Read the model definition and answer for the solid it produces. Units are mm, in the model's axes. A direction names the side the tool comes from. Coordinates: 2 decimals unless noted, no trailing zeros. Order: outer loops, then holes, each group sorted by start corner. A loop starts at its lowest first (then second) coordinate and runs counter-clockwise, first axis right, second up. Notation, with made-up numbers: (32.5, -2) -> (65.5, -2) arc R20 cw to (65.5, 23) -> close; hole circle Ø6 at (88.25, 57). An arc over 180 degrees is marked (long way). Answer in a Markdown table with one row per item.
from build123d import *

# Parameters (mm, degrees)
SKETCH1_R           = 28.575
SKETCH1_R_2         = 2.54
BOSS_EXTRUDE1_DEPTH = 4.064
SKETCH2_R           = 14.2875
BOSS_EXTRUDE2_DEPTH = 0.8636
SKETCH3_R           = 12.065
EXTRUDE_M_DEPTH     = 20.4724


with BuildPart() as part:
    # Sketch1 → Boss-Extrude1 (new body)
    with BuildSketch(Plane.XY):
        Circle(SKETCH1_R)
        with Locations((0, 23.8125)):
            Circle(SKETCH1_R_2, mode=Mode.SUBTRACT)
        with Locations((20.622229928, 11.90625)):
            Circle(SKETCH1_R_2, mode=Mode.SUBTRACT)
        with Locations((20.622229928, -11.90625)):
            Circle(SKETCH1_R_2, mode=Mode.SUBTRACT)
        with Locations((0, -23.8125)):
            Circle(SKETCH1_R_2, mode=Mode.SUBTRACT)
        with Locations((-20.622229928, -11.90625)):
            Circle(SKETCH1_R_2, mode=Mode.SUBTRACT)
        with Locations((-20.622229928, 11.90625)):
            Circle(SKETCH1_R_2, mode=Mode.SUBTRACT)
        Polygon((7.332348419, 0), (3.666174209, 6.35), (-3.666174209, 6.35), (-7.332348419, 0), (-3.666174209, -6.35), (3.666174209, -6.35), align=None, mode=Mode.SUBTRACT)
    extrude(amount=BOSS_EXTRUDE1_DEPTH)

    # Sketch2 → Boss-Extrude2 (add)
    with BuildSketch(Plane.XY.offset(4.064)):
        Circle(SKETCH2_R)
        Polygon((-3.666174209, 6.35), (3.666174209, 6.35), (7.332348419, 0), (3.666174209, -6.35), (-3.666174209, -6.35), (-7.332348419, 0), align=None, mode=Mode.SUBTRACT)
    extrude(amount=BOSS_EXTRUDE2_DEPTH)

    # Sketch3 → Extrude m (add)
    with BuildSketch(Plane(origin=(0, 0, 0), x_dir=(-1, 0, 0), z_dir=(0, 0, -1))):
        with Locations(Location((0, 0, 0), (0, 0, 180))):
            Circle(SKETCH3_R)
        Polygon((7.332348419, 0), (3.666174209, 6.35), (-3.666174209, 6.35), (-7.332348419, 0), (-3.666174209, -6.35), (3.666174209, -6.35), align=None, mode=Mode.SUBTRACT)
    extrude(amount=EXTRUDE_M_DEPTH)


solid = part.part
Q1. The part is cut by section D-D (x = -20). Write down the section's boundary in (y, z), then the cut area to 3 significant figures.
Outcome:
| item | result |
|---|---|
| outline | (-20.41, 0) -> (-14.37, 0) -> (-14.37, 4.06) -> (-20.41, 4.06) -> close; (-9.44, 0) -> (9.44, 0) -> (9.44, 4.06) -> (-9.44, 4.06) -> close; (14.37, 0) -> (20.41, 0) -> (20.41, 4.06) -> (14.37, 4.06) -> close |
| area | 126 mm² |
Q2. Consider line 1 (X direction, y = -13.5, z = 3.75); line 2 (Z direction, x = 18.5, y = -4); line 3 (Y direction, x = 11, z = 3). Determine where each line is inside the solid, lowest interval first.
Outcome:
| item | result |
|---|---|
| line 1 | -25.18 to -22.6, -18.64 to 18.64, 22.6 to 25.18 |
| line 2 | 0 to 4.06 |
| line 3 | -26.37 to 26.37 |
Q3. For a pull along Y with two mould halves and no side action, classify faces 1 (the face through (5, 5, -20.472)), 2 (the face through (-5.474, -3.219, -7.595)), 3 (the face through (-5.525, 3.131, -7.595)), 4 (the face through (-14.274, 0.628, 4.49)) as pulls with the +Y half, pulls with the -Y half, needs draft (parallel to the pull), parting line crosses it, or undercut.
Outcome:
| item | result |
|---|---|
| face 1 | needs draft |
| face 2 | undercut |
| face 3 | undercut |
| face 4 | parting line crosses it |
Q4. Given pin 1 (2 mm diameter, centred on x = 0, z = -12, fed in from +Y) (3 decimals); pin 2 (1.5 mm diameter, centred on x = 19.5, z = 0.5, fed in from -Y); pin 3 (6 mm diameter, centred on x = 20.62, y = -11.91, fed in from -Z); pin 4 (17 mm diameter, centred on x = 0, y = -5, fed in from -Z), each flat-ended and moving along its own axis, determine where each tip first touches the part or whether it passes through.
Outcome:
| item | result |
|---|---|
| pin 1 | y = 12.065 |
| pin 2 | y = -21.56 |
| pin 3 | z = 0 |
| pin 4 | z = -20.47 |
Q5. For faces 5 (the face through (0, 6.35, -8)), 6 (the face through (11.51, -3.62, -10.09)), 7 (the face through (-13, 7, 4.064)), 8 (the face through (0, 7, 4.928)), determine the directions among +Z, -Z, +X, -X, +Y, -Y from which every point of the face is accessible in a straight line to the end or side of a thin tool.
Outcome:
| item | result |
|---|---|
| face 5 | +Z, -Z |
| face 6 | -Z |
| face 7 | +Z |
| face 8 | +Z, +X, -X, +Y, -Y |
Q6. The part is cut by section B-B (y = 22). Write down the section's boundary in (x, z), then the cut area to 3 significant figures.
Outcome:
| item | result |
|---|---|
| outline | (-18.24, 0) -> (-1.78, 0) -> (-1.78, 4.06) -> (-18.24, 4.06) -> close; (1.78, 0) -> (18.24, 0) -> (18.24, 4.06) -> (1.78, 4.06) -> close |
| area | 134 mm² |
Q7. The part is cut by section C-C (z = -9). Write down the section's boundary in (x, y) (3 decimals), then the cut area to 3 significant figures.
Outcome:
| item | result |
|---|---|
| outline | circle Ø24.13 at (0, 0); hole (-7.332, 0) -> (-3.666, -6.35) -> (3.666, -6.35) -> (7.332, 0) -> (3.666, 6.35) -> (-3.666, 6.35) -> close |
| area | 318 mm² |
Q8. The part is cut by section A-A (x = 0). Give the number of separate pieces and of enclosed holes in the cut face, then the cut area to 3 significant figures.
Outcome:
| item | result |
|---|---|
| separate pieces | 4 |
| enclosed holes | 0 |
| area | 387 mm² |
